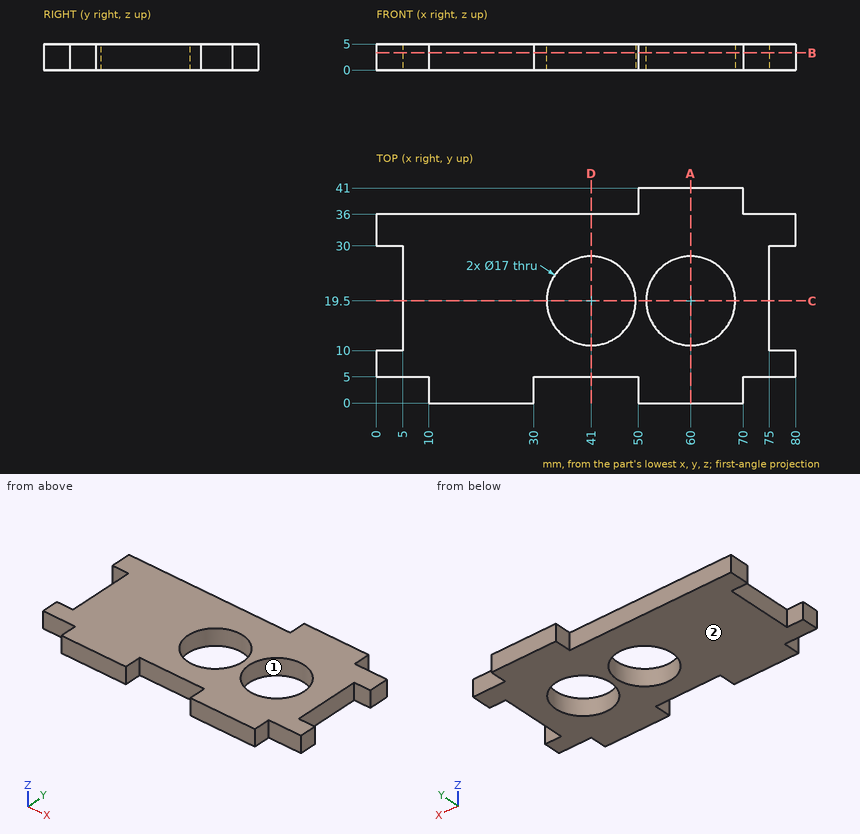
Study the drawing (mm; zero at the part's minimum x, y, z) and answer. Give positions to 0.01 mm unless a question says otherwise; leave off trailing zeros. Write each loop counter-clockwise with the first axis right and the second up, starting at its lowest first coordinate (ties: lowest second). Pieces come first, ordered by that corner, then holes. Notation, with made-up numbers: (16, -37) - (67, -37) arc R16 cw to (67, -9) - close; hole circle Ø3 at (23.25, 40). An arc over 180 degrees is marked (long way). Use CSV: the item, a comma, the result in double quotes. Start each with the question number.
(1) Find section C-C (y = 19.5). Give the vertices of the cut face in (x, z).
(2) Consider line 1 along Y through (x, z) = (60, 1.2); line 2 along Y through (x, z) = (41, 2.4); line 3 along Y through (x, z) = (20, 4.05). Determine where each line is inside the solid, lowest interval first.
(3) Find section B-B (z = 3.3). Give the vertices of the cut face in (x, y).
(4) Given P1, Ø2.5, axis at y = 20, z = 3, coming from the -X side; P2, Ø1.5, axis at y = 39.5, z = 3, coming from the -X side; P3, Ø1.5, axis at y = 18.5, z = 3.5, coming from the +X side, each flat-ended and moving along its own axis, determine where each tip first touches the part or whether it passes through.
(5) Determine the mould class of the marked faces 1 and 2 for opening direction Y: +Y half, -Y half, draft (parallel to the pull), parting line (faces both ways), or undercut.
(6) Find section A-A (x = 60). Give the vertices of the cut face in (y, z), plus the area to 3 significant figures.
(7) Find section D-D (x = 41). Give the vertices of the cut face in (y, z).
Findings below:
1,outline,"(5, 0) - (32.5, 0) - (32.5, 5) - (5, 5) - close; (49.5, 0) - (51.5, 0) - (51.5, 5) - (49.5, 5) - close; (68.5, 0) - (75, 0) - (75, 5) - (68.5, 5) - close"
2,line 1,"0 to 11, 28 to 41"
2,line 2,"5 to 11, 28 to 36"
2,line 3,"0 to 36"
3,outline,"(0, 5) - (10, 5) - (10, 0) - (30, 0) - (30, 5) - (50, 5) - (50, 0) - (70, 0) - (70, 5) - (80, 5) - (80, 10) - (75, 10) - (75, 30) - (80, 30) - (80, 36) - (70, 36) - (70, 41) - (50, 41) - (50, 36) - (0, 36) - (0, 30) - (5, 30) - (5, 10) - (0, 10) - close; hole circle Ø17 at (41, 19.5); hole circle Ø17 at (60, 19.5)"
4,P1,"x = 5"
4,P2,"x = 50"
4,P3,"x = 75"
5,face 1,"undercut"
5,face 2,"draft"
6,outline,"(0, 0) - (11, 0) - (11, 5) - (0, 5) - close; (28, 0) - (41, 0) - (41, 5) - (28, 5) - close"
6,area,"120 mm2"
7,outline,"(5, 0) - (11, 0) - (11, 5) - (5, 5) - close; (28, 0) - (36, 0) - (36, 5) - (28, 5) - close"
